```python
from build123d import *

# Parameters (mm, degrees)
F1_DEPTH = 60
F2_DEPTH = 20
F4_DEPTH = 100.001
F6_DEPTH = 60.001


with BuildPart() as f1:
    # F0 (on Top) → F1 (new body)
    with BuildSketch(Plane.XY):
        Polygon((0, 40), (0, 0), (20, 0), (20, 15), (55, 15), (55, 0), (70, 0), (70, 20), (100, 20), (100, 40), align=None)
    extrude(amount=F1_DEPTH)

    # F2 (add): a face of the model
    f2_faces = [f1.faces().sort_by_distance(p)[0] for p in [
        (50, 40, 30),
    ]]
    extrude(f2_faces, amount=F2_DEPTH)

    # F3 (on Right) → F4 (cut, through all)
    with BuildSketch(Plane.YZ):
        Polygon((50, 60), (20, 60), (0, 60), (0, 5), align=None)
    extrude(amount=F4_DEPTH, mode=Mode.SUBTRACT)

    # F5 (on Front) → F6 (cut, through all)
    with BuildSketch(Plane.XZ):
        Polygon((0, 60), (0, 40), (4.0449425578, 40), (38.6859587092, 60), align=None)
        Polygon((100, 60), (79.9438208342, 60), (100, 39.9438208342), align=None)
    extrude(amount=-F6_DEPTH, mode=Mode.SUBTRACT)


solid = f1.part
```
Input: part model. Units: mm. Frame: model coordinates. A direction names the side the tool comes from. Round coordinates to 2 decimals unless told otherwise and drop trailing zeros. Loops run counter-clockwise (first coordinate to the right, second up) from the corner with the lowest first, then second, coordinate; pieces in that order, holes last. Notation, with made-up numbers: (77, 41) -> (135, 41) arc R27 cw to (135, 74) -> close; hole circle Ø11 at (65.25, -36). An arc over 180 degrees is marked (long way). One line per item, written item: value.
(1) Pin query (flat end, axial travel): pin 1 (5 mm diameter, centred on x = 41.5, z = 18, fed in from -Y); pin 2 (16.5 mm diameter, centred on y = 5, z = 9, fed in from -X); pin 3 (16 mm diameter, centred on y = 11, z = 8, fed in from +X); pin 4 (8 mm diameter, centred on x = 77.5, z = 19, fed in from -Y). Return the tip coordinate at first contact, or that it passes through.
Geometry check:
pin 1: y = 15
pin 2: x = 0
pin 3: x = 70
pin 4: y = 20
(2) Section A-A (y = 7). Return the cut outline in (x, z).
Geometry check:
outline: (0, 0) -> (20, 0) -> (20, 12.7) -> (0, 12.7) -> close; (55, 0) -> (70, 0) -> (70, 12.7) -> (55, 12.7) -> close
(3) Section D-D (z = 15). Return the cut outline in (x, y), plus the area to 3 significant figures.
Geometry check:
outline: (0, 9.09) -> (20, 9.09) -> (20, 15) -> (55, 15) -> (55, 9.09) -> (70, 9.09) -> (70, 20) -> (100, 20) -> (100, 60) -> (0, 60) -> close
area: 4,560 mm2
(4) Mould query, pull axis X, two halves, no side actions, for faces 5 (the face through (60, 55, 60)), 6 (the face through (55, 9, 8)), 7 (the face through (37, 15, 11)), 8 (the face through (17.274, 48.843, 47.638)). Classes: pulls with the +X half, pulls with the -X half, needs draft (parallel to the pull), parting line crosses it, or undercut.
Geometry check:
face 5: needs draft
face 6: undercut
face 7: undercut
face 8: pulls with the -X half
(5) Material intervals for line 1 (Y direction, x = 79, z = 24.5); line 2 (X direction, y = 10.5, z = 8.5); line 3 (Y direction, x = 49, z = 20), sorted ascending. Write a range as [from, to].
Geometry check:
line 1: [20, 60]
line 2: [0, 20], [55, 70]
line 3: [15, 60]
(6) Set-up query: faces 1 (the face through (51, 60, 30)), 2 (the face through (20, 9, 8)), 3 (the face through (2, 46, 40)), 4 (the face through (85, 20, 13)). Return all of +Z, -Z, +X, -X, +Y, -Y with unobstructed straight access to the full face (end or side cutting, diameter ignored); none if empty.
Geometry check:
face 1: +Z, -Z, +X, -X, +Y
face 2: +Z, -Z, -Y
face 3: +Z, -X, +Y, -Y
face 4: +Z, -Z, +X, -Y
(7) Section C-C (y = 56). Return the cut outline in (x, z).
Geometry check:
outline: (0, 0) -> (100, 0) -> (100, 39.94) -> (79.94, 60) -> (38.69, 60) -> (4.04, 40) -> (0, 40) -> close
(8) Section B-B (x = 76). Return the cut outline in (y, z), plus the area to 4 significant figures.
Geometry check:
outline: (20, 0) -> (60, 0) -> (60, 60) -> (50, 60) -> (20, 27) -> close
area: 1,905 mm2
